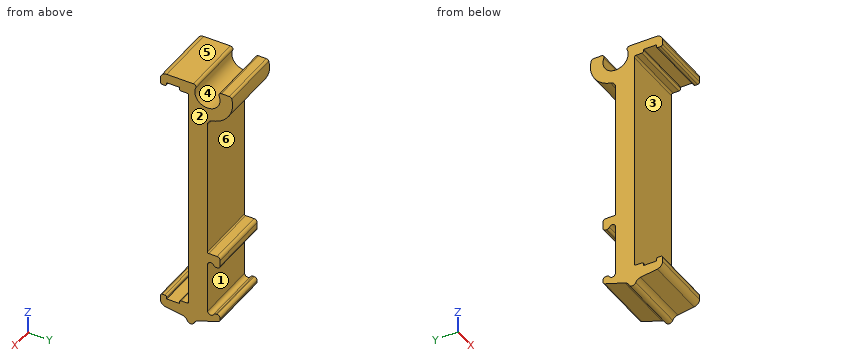
```python
from build123d import *

# Parameters (mm, degrees)
F3_DEPTH = 10


with BuildPart() as f3:
    # F2 (on Right) → F3 (new body)
    with BuildSketch(Plane.YZ):
        with BuildLine():
            ThreePointArc((-4.5, 35.8), (-4.412132, 35.587868), (-4.2, 35.5))
            Line((-4.2, 35.5), (-3.8, 35.5))
            ThreePointArc((-3.8, 35.5), (-3.587868, 35.587868), (-3.5, 35.8))
            Line((-3.5, 35.8), (-3.5, 36.05))
            Line((-3.5, 36.05), (-1.5, 36.05))
            Line((-1.5, 36.05), (-1.5, 35.8))
            ThreePointArc((-1.5, 35.8), (-1.412132, 35.587868), (-1.2, 35.5))
            Line((-1.2, 35.5), (-0.3, 35.5))
            ThreePointArc((-0.3, 35.5), (-0.087868, 35.412132), (0, 35.2))
            Line((0, 35.2), (0, -0.2))
            ThreePointArc((0, -0.2), (-0.087868, -0.412132), (-0.3, -0.5))
            Line((-0.3, -0.5), (-1.2, -0.5))
            ThreePointArc((-1.2, -0.5), (-1.412132, -0.587868), (-1.5, -0.8))
            Line((-1.5, -0.8), (-1.5, -1.05))
            Line((-1.5, -1.05), (-3.5, -1.05))
            Line((-3.5, -1.05), (-3.5, -0.8))
            ThreePointArc((-3.5, -0.8), (-3.587868, -0.587868), (-3.8, -0.5))
            Line((-3.8, -0.5), (-4.2, -0.5))
            ThreePointArc((-4.2, -0.5), (-4.412132, -0.587868), (-4.5, -0.8))
            Line((-4.5, -0.8), (-4.5, -1.5))
            ThreePointArc((-4.5, -1.5), (-4.257206, -2.153176), (-3.646721, -2.489178))
            Line((-3.646721, -2.489178), (-1.020876, -2.87866))
            ThreePointArc((-1.020876, -2.87866), (-0.55385, -3.078335), (-0.245161, -3.481689))
            ThreePointArc((-0.245161, -3.481689), (0.31218, -3.849987), (0.864712, -3.474515))
            ThreePointArc((0.864712, -3.474515), (1.107187, -3.120048), (1.47598, -2.899975))
            Line((1.47598, -2.899975), (4.658042, -1.839826))
            ThreePointArc((4.658042, -1.839826), (4.905599, -1.657846), (5, -1.36546))
            Line((5, -1.36546), (5, -1.145353))
            ThreePointArc((5, -1.145353), (4.853553, -0.7918), (4.5, -0.645353))
            Line((4.5, -0.645353), (4.366025, -0.645353))
            ThreePointArc((4.366025, -0.645353), (4.116025, -0.71234), (3.933013, -0.895353))
            ThreePointArc((3.933013, -0.895353), (3.37059, -1.128316), (3, -0.645353))
            Line((3, -0.645353), (3, 7.354647))
            ThreePointArc((3, 7.354647), (3.37059, 7.83761), (3.933013, 7.604647))
            ThreePointArc((3.933013, 7.604647), (4.116025, 7.421634), (4.366025, 7.354647))
            Line((4.366025, 7.354647), (4.5, 7.354647))
            ThreePointArc((4.5, 7.354647), (4.853553, 7.501094), (5, 7.854647))
            Line((5, 7.854647), (5, 8.801021))
            ThreePointArc((5, 8.801021), (4.853553, 9.154574), (4.5, 9.301021))
            Line((4.5, 9.301021), (3.168028, 9.301021))
            ThreePointArc((3.168028, 9.301021), (3.026607, 9.359599), (2.968028, 9.501021))
            Line((2.968028, 9.501021), (2.968028, 31.301021))
            ThreePointArc((2.968028, 31.301021), (3.193432, 31.933476), (3.768028, 32.280816))
            ThreePointArc((3.768028, 32.280816), (6.360488, 34.080751), (6.841012, 37.2))
            ThreePointArc((6.841012, 37.2), (6.698662, 37.416228), (6.453713, 37.5))
            Line((6.453713, 37.5), (5.192888, 37.5))
            ThreePointArc((5.192888, 37.5), (4.861225, 37.323607), (4.822078, 36.95))
            ThreePointArc((4.822078, 36.95), (2.968028, 34.2), (1.113979, 36.95))
            ThreePointArc((1.113979, 36.95), (1.074831, 37.323607), (0.743169, 37.5))
            Line((0.743169, 37.5), (-3.5, 37.5))
            ThreePointArc((-3.5, 37.5), (-4.207107, 37.207107), (-4.5, 36.5))
            Line((-4.5, 36.5), (-4.5, 35.8))
        make_face()
    extrude(amount=F3_DEPTH)


solid = f3.part
```
Geometry: final body of the model. Coordinates: model frame, mm. Face numbers are marked on the shaded views. A direction names the side the tool comes from. Coordinates: 2 decimals unless noted, no trailing zeros. Loops run counter-clockwise (first coordinate to the right, second up) from the corner with the lowest first, then second, coordinate; pieces in that order, holes last. Notation, with made-up numbers: (22, 46) -> (40, 46) arc R30 cw to (40, 85) -> close; hole circle Ø10 at (-28, -36.5). An arc over 180 degrees is marked (long way). Use a Markdown table: item, result. Add a question column.
(1) Mould query, pull axis Y, two halves, no side actions, for the marked faces 4, 5 and 6. Classes: pulls with the +Y half, pulls with the -Y half, needs draft (parallel to the pull), parting line crosses it, or undercut.
(2) Access query for the marked faces 1, 2 and 3. Directions: +Z, -Z, +X, -X, +Y, -Y. A direction counts if a zero-diameter tool reaches every point of the face in a straight line with its end or side. Return the directions, or none.
(3) Line query: line 1 along Y through (x, z) = (7, 36.2); line 2 along Z through (x, y) = (8.75, 3.75); line 3 along Z through (x, y) = (0.5, 3.5). Output: solid intervals per line, ascending.
(4) Section query B-B, the plane z = 1. Return loops of the section in (x, y).
(5) Section query A-A, the plane z = 29.5. Return loops of the section in (x, y), plus the area to 3 significant figures.
(6) Pin query (flat end, axial travel): pin 1 Ø5 at (x, z) = (5.5, 15) entering from +Y; pin 2 Ø0.6 at (x, y) = (7.5, -2.5) entering from -Z; pin 3 Ø6 at (y, z) = (5, 31.5) entering from +X; pin 4 Ø0.7 at (x, y) = (4.5, 3.5) entering from +Z (3 decimals). Return the tip coordinate at first contact, or that it passes through.
Answer:
| question | item | result |
|---|---|---|
| 1 | face 4 | undercut |
| 1 | face 5 | needs draft |
| 1 | face 6 | pulls with the +Y half |
| 2 | face 1 | +X, -X, +Y |
| 2 | face 2 | +Z, -Z, +X, +Y, -Y |
| 2 | face 3 | +X, -X, -Y |
| 3 | line 1 | y = -4.5 to 0.97, 4.97 to 6.97 |
| 3 | line 2 | z = -2.14 to -1.08, 7.79 to 9.3, 32.28 to 34.36 |
| 3 | line 3 | z = -2.23 to -1.15, 7.85 to 9.3, 32.18 to 34.27 |
| 4 | outline | (0, 0) -> (10, 0) -> (10, 3) -> (0, 3) -> close |
| 5 | outline | (0, 0) -> (10, 0) -> (10, 2.97) -> (0, 2.97) -> close |
| 5 | area | 29.7 mm^2 |
| 6 | pin 1 | stops at y = 2.97 |
| 6 | pin 2 | stops at z = -2.7 |
| 6 | pin 3 | stops at x = 10 |
| 6 | pin 4 | stops at z = 34.405 |
